The model under review builds one solid part; all positions refer to its coordinate system, in mm. Face numbers are marked on the shaded views. Coordinates: 2 decimals unless noted, no trailing zeros. Loops run counter-clockwise (first coordinate to the right, second up) from the corner with the lowest first, then second, coordinate; pieces in that order, holes last. Notation, with made-up numbers: (54.25, 54.5) - (73.25, 54.5) arc R32 ccw to (73.25, 83.5) - close; hole circle Ø7 at (49, 35.5). An arc over 180 degrees is marked (long way). Answer in a Markdown table with one row per item. Add a question column.
(1) We need section B-B on x = -9.5. Write out the cut boundary in (y, z).
(2) For line 1 along X through (y, z) = (1.5, 3.5); line 2 along Z through (x, y) = (-2.75, 1.75); line 3 along X through (y, z) = (0.5, -0.25), list the stretches that pass through material, from the lowest coordinate up.
(3) Mouldability with a two-part tool opening along Y and no side actions: class the marked faces 1, 2 and 3 as +Y half, -Y half, draft (parallel to the pull), parting line (faces both ways), or undercut.
(4) We need section C-C on x = -4.5. Write out the cut boundary in (y, z), plus the area to 3 significant figures.
(5) We need section A-A on x = -1.75. Write out the cut boundary in (y, z).
(6) For P1, Ø4, axis at y = 0, z = 0, coming from the +X side; P2, Ø1.5, axis at x = -8.5, z = 1, coming from the -Y side; P3, Ø2, axis at x = -8.5, z = 2, coming from the +Y side; P4, Ø4, axis at y = 1, z = -1.5, coming from the -X side, all flat-tipped, find the tip position at first contact; note any pin that passes through.
from build123d import *

# Parameters (mm, degrees)
SKETCH_2_R          = 2.5
CUT_EXTRUDE_1_DEPTH = 3.5
SKETCH_3_R          = 1.5
CUT_EXTRUDE_2_DEPTH = 1
FILLET_1_R          = 0.2
SKETCH_4_R          = 0.05
EXTRUDE_1_DEPTH     = 0.05


with BuildPart() as part:
    # 草图1 → 旋转1 (revolve)
    with BuildSketch(Plane.XY, mode=Mode.PRIVATE) as revolve_1_sk:
        Polygon((0, 0), (0, 4), (-0.3, 4), (-0.3, 3.7), (-15, 0.5), (-15, 0), align=None)
    revolve(revolve_1_sk.sketch.rotate(Axis((-15, 0, 0), (1, 0, 0)), 90), axis=Axis((-15, 0, 0), (1, 0, 0)))

    # 草图2 → 切除-拉伸1 (cut)
    with BuildSketch(Plane(origin=(0, 0, 0), x_dir=(0, 0, -1), z_dir=(1, 0, 0))):
        Circle(SKETCH_2_R)
    extrude(amount=-CUT_EXTRUDE_1_DEPTH, mode=Mode.SUBTRACT)

    # 草图3 → 切除-拉伸2 (cut)
    with BuildSketch(Plane.ZY.offset(15)):
        Circle(SKETCH_3_R)
    extrude(amount=-CUT_EXTRUDE_2_DEPTH, mode=Mode.SUBTRACT)

    # 圆角1
    fillet_1_edges = [part.edges().sort_by_distance(p)[0] for p in [
        (-14, 0, -0.717687075),
    ]]
    fillet(fillet_1_edges, radius=FILLET_1_R)

    # 草图4 → 凸台-拉伸1 (add)
    with BuildSketch(Plane.ZY.offset(14)):
        Circle(SKETCH_4_R)
    extrude(amount=EXTRUDE_1_DEPTH)

    # 草图5 → 切除-旋转1 (revolve, cut)
    with BuildSketch(Plane(origin=(0, 0, 0), x_dir=(1, 0, 0), z_dir=(0, 1, 0)), mode=Mode.PRIVATE) as cut_revolve_1_sk:
        Polygon((-14, -0.05), (-14.05, -0.03), (-14.05, -0.05), align=None)
    revolve(cut_revolve_1_sk.sketch.rotate(Axis((-14.05, 0, 0), (1, 0, 0)), 180), axis=Axis((-14.05, 0, 0), (1, 0, 0)), mode=Mode.SUBTRACT)


solid = part.part
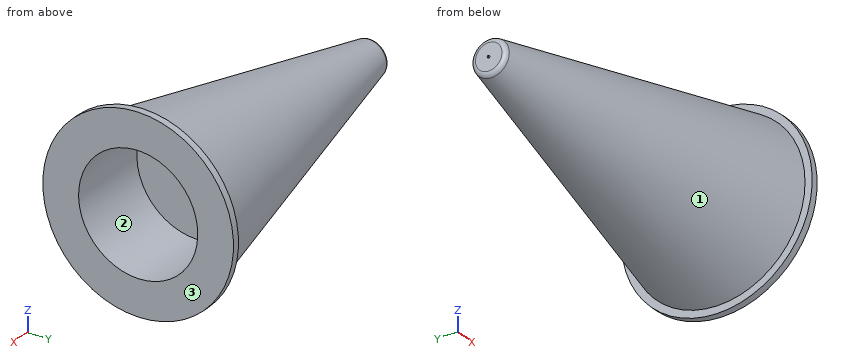
Outcome:
| question | item | result |
|---|---|---|
| 1 | outline | circle Ø3.39 at (0, 0) |
| 2 | line 1 | -0.3 to 0 |
| 2 | line 2 | -2.64 to -1.79, 1.79 to 2.64 |
| 2 | line 3 | -14 to -3.5 |
| 3 | face 1 | parting line |
| 3 | face 2 | undercut |
| 3 | face 3 | draft |
| 4 | outline | circle Ø5.57 at (0, 0) |
| 4 | area | 24.4 mm² |
| 5 | outline | circle Ø6.77 at (0, 0); hole circle Ø5 at (0, 0) |
| 6 | P1 | x = -3.5 |
| 6 | P2 | y = -1.98 |
| 6 | P3 | y = 1.68 |
| 6 | P4 | x = -14.05 |
